```python
from build123d import *

# Parameters (mm, degrees)
SKETCH1_W               = 50
SKETCH1_H               = 95
BOSS_EXTRUDE1_DEPTH     = 4.5
SKETCH2_R               = 0.5
CUT_EXTRUDE1_DEPTH      = 108.448825028
SKETCH3_W               = 2
SKETCH3_H               = 2.25
CUT_EXTRUDE2_DEPTH      = 108.448825028
SKETCH5_R               = 2.5
BOSS_EXTRUDE2_DEPTH     = 2
SKETCH6_R               = 1.5
CUT_EXTRUDE3_DEPTH      = 108.551150621
FILLET1_R               = 4
SKETCH8_W               = 5.5
SKETCH8_H               = 30
CUT_EXTRUDE4_DEPTH      = 3
SKETCH10_W              = 2
SKETCH10_H              = 2.25
CUT_EXTRUDE5_DEPTH      = 4.5
FILLET2_R               = 1
SKETCH11_W              = 8
SKETCH11_H              = 2
BOSS_EXTRUDE3_DEPTH     = 8
CUT_EXTRUDE6_DEPTH      = 109.079831606
CUT_EXTRUDE6_DEPTH_BACK = 109.079831606
SKETCH12_R              = 1.7
FILLET3_R               = 2


with BuildPart() as part:
    # Sketch1 → Boss-Extrude1 (new body)
    with BuildSketch(Plane(origin=(0, 0, 0), x_dir=(0, 1, 0), z_dir=(0, 0, 1))):
        with Locations((25, 47.5)):
            Rectangle(SKETCH1_W, SKETCH1_H)
    extrude(amount=BOSS_EXTRUDE1_DEPTH)

    # Sketch2 → Cut-Extrude1 (cut, through all)
    with BuildSketch(Plane.XY.offset(4.5)):
        with Locations((-60, 25)):
            Circle(SKETCH2_R)
    extrude(amount=-CUT_EXTRUDE1_DEPTH, mode=Mode.SUBTRACT)

    # Sketch3 → Cut-Extrude2 (cut, through all)
    with BuildSketch(Plane(origin=(-95, 0, 0), x_dir=(0, -1, 0), z_dir=(-1, 0, 0))):
        with Locations((-49, 1.125)):
            Rectangle(SKETCH3_W, SKETCH3_H)
        with Locations((-1, 1.125)):
            Rectangle(SKETCH3_W, SKETCH3_H)
    extrude(amount=-CUT_EXTRUDE2_DEPTH, mode=Mode.SUBTRACT)

    # Sketch5 → Boss-Extrude2 (add)
    with BuildSketch(Plane.XY.offset(4.5)):
        with Locations(Location((-60, 25, 0), (0, 0, 180))):
            Circle(SKETCH5_R)
    extrude(amount=BOSS_EXTRUDE2_DEPTH)

    # Sketch6 → Cut-Extrude3 (cut, through all)
    with BuildSketch(Plane.XY.offset(6.5)):
        with Locations((-60, 25)):
            Circle(SKETCH6_R)
    extrude(amount=-CUT_EXTRUDE3_DEPTH, mode=Mode.SUBTRACT)

    # Fillet1
    # the kernel refuses this fillet: 4 mm, written as the material it adds along each edge
    with BuildSketch(Plane(origin=(-60, 25, 4.5), x_dir=(-1, 0, 0), z_dir=(0, 1, 0))) as fillet1_piece_1:
        with BuildLine():
            CenterArc((5.964101615, 4), FILLET1_R, 210, 60)
            Line((2.5, 2), (2.430717968, 1.96))
            ThreePointArc((2.430717968, 1.96), (2.42, 1), (2.42, 0))
            Line((2.42, 0), (2.5, -0.08))
            Line((2.5, -0.08), (5.964101615, -0.08))
            Line((5.964101615, -0.08), (5.964101615, 0))
        make_face()
    revolve(axis=Axis((-60, 25, 4.5), (0, 0, 1)))

    # Sketch8 → Cut-Extrude4 (cut)
    with BuildSketch(Plane(origin=(0, 0, 0), x_dir=(1, 0, 0), z_dir=(0, 0, -1))):
        with Locations((-60, -35)):
            Rectangle(SKETCH8_W, SKETCH8_H)
    extrude(amount=-CUT_EXTRUDE4_DEPTH, mode=Mode.SUBTRACT)

    # Sketch10 → Cut-Extrude5 (cut)
    with BuildSketch(Plane(origin=(-95, 0, 0), x_dir=(0, -1, 0), z_dir=(-1, 0, 0))):
        with Locations((-49, 3.375)):
            Rectangle(SKETCH10_W, SKETCH10_H)
        with Locations((-1, 3.375)):
            Rectangle(SKETCH10_W, SKETCH10_H)
    extrude(amount=-CUT_EXTRUDE5_DEPTH, mode=Mode.SUBTRACT)

    # Fillet2
    fillet2_edges = [part.edges().sort_by_distance(p)[0] for p in [
        (-95, 25, 0),
        (-95, 48, 2.25),
        (-95, 2, 2.25),
    ]]
    fillet(fillet2_edges, radius=FILLET2_R)

    # Sketch11 → Boss-Extrude3 (add)
    with BuildSketch(Plane.XY.offset(4.5)):
        with Locations((-4, 49)):
            Rectangle(SKETCH11_W, SKETCH11_H)
        with Locations((-4, 1)):
            Rectangle(SKETCH11_W, SKETCH11_H)
    extrude(amount=BOSS_EXTRUDE3_DEPTH)

    # Sketch12 → Cut-Extrude6 (cut, two sides: drawn at the far end of the back side and taken through both)
    with BuildSketch(Plane(origin=(0, 50, 0), x_dir=(-1, 0, 0), z_dir=(0, 1, 0)).offset(-CUT_EXTRUDE6_DEPTH_BACK)):
        with Locations((4, 8.5)):
            Circle(SKETCH12_R)
    extrude(amount=CUT_EXTRUDE6_DEPTH + CUT_EXTRUDE6_DEPTH_BACK, mode=Mode.SUBTRACT)

    # Fillet3
    fillet3_edges = [part.edges().sort_by_distance(p)[0] for p in [
        (-8, 49, 4.5),
        (0, 49, 12.5),
        (-8, 49, 12.5),
        (-8, 1, 4.5),
        (0, 1, 12.5),
        (-8, 1, 12.5),
    ]]
    fillet(fillet3_edges, radius=FILLET3_R)


solid = part.part
```
Input: part model. Units: mm. Frame: model coordinates. A direction names the side the tool comes from. Round coordinates to 2 decimals unless told otherwise and drop trailing zeros. Loops run counter-clockwise (first coordinate to the right, second up) from the corner with the lowest first, then second, coordinate; pieces in that order, holes last. Notation, with made-up numbers: (58, 40) - (110, 40) arc R21 cw to (110, 60) - close; hole circle Ø10 at (-30.5, 56.25). An arc over 180 degrees is marked (long way). One line per item, written item: value. Start each with the question number.
(1) Ray query, line 1 (Z direction, x = -4, y = 0.5); line 2 (X direction, y = 1.3, z = 8.5); line 3 (Z direction, x = -74.5, y = 29). Return the intervals inside material, ascending. Write a range as [from, to].
(2) Section A-A, the plane x = -4. Return loops of the section in (y, z), plus the area to 3 significant figures.
(3) Section C-C, the plane y = 25. Return loops of the section in (x, z), plus the area to 3 significant figures.
(4) Access query for faces 5 (the flat face through (-8, 49, 8)), 6 (the flat face through (-5.1, 2, 6.7)), 7 (the flat face through (-39, 50, 4)), 8 (the flat face through (-60, 20, 1)), 9 (the flat face through (-90.5, 49, 3)). Directions: +Z, -Z, +X, -X, +Y, -Y. A direction counts if a zero-diameter tool reaches every point of the face in a straight line with its end or side. Return the directions, or none.
(5) Draft query along X for faces 1 (the flat face through (-57.25, 35, 1)), 2 (the flat face through (-62.75, 35, 1)), 3 (the flat face through (-29, 48, 1)), 4 (the cylindrical face through (-0.57, 1.01, 11.9)). Return one class per face: +X half, -X half, draft (parallel to the pull), parting line (faces both ways), or undercut.
(6) Section B-B, the plane z = 8.5. Return loops of the section in (x, y), plus the area to 3 significant figures.
(7) Section D-D, the plane x = -71.5. Return loops of the section in (y, z).
(8) Contact query for flat-ended pins moving along their axis: P1, Ø1, axis at y = 49, z = 3.5, coming from the -X side; P2, Ø0.7, axis at x = -40.5, z = 1.5, coming from the +Y side; P3, Ø2, axis at y = 1, z = 9, coming from the -X side. Output: stop coordinate, or through.
Results below:
1. line 1: [2.25, 6.8], [10.2, 12.5]
1. line 2: [-8, -5.7], [-2.3, 0]
1. line 3: [0, 4.5]
2. outline: (0, 2.25) - (2, 2.25) - (2, 0) - (48, 0) - (48, 2.25) - (50, 2.25) - (50, 6.8) - (48, 6.8) - (48, 4.5) - (2, 4.5) - (2, 6.8) - (0, 6.8) - close; (0, 10.2) - (2, 10.2) - (2, 12.5) - (0, 12.5) - close; (48, 10.2) - (50, 10.2) - (50, 12.5) - (48, 12.5) - close
2. area: 234 mm^2
3. outline: (-95, 1) arc R1 ccw to (-94, 0) - (-62.75, 0) - (-62.75, 3) - (-61.5, 3) - (-61.5, 6.5) - (-62.5, 6.5) arc R4 cw to (-65.96, 4.5) - (-95, 4.5) - close; (-58.5, 3) - (-57.25, 3) - (-57.25, 0) - (0, 0) - (0, 4.5) - (-54.04, 4.5) arc R4 cw to (-57.5, 6.5) - (-58.5, 6.5) - close
3. area: 414 mm^2
4. face 5: +Z, -X, +Y, -Y
4. face 6: +Z, +X, -X
4. face 7: +Z, -Z, +X, -X, +Y
4. face 8: -Z, +Y
4. face 9: +Z, -Z, -X, +Y
5. face 1: undercut
5. face 2: undercut
5. face 3: draft
5. face 4: +X half
6. outline: (-8, 0) - (-5.7, 0) - (-5.7, 2) - (-8, 2) - close; (-8, 48) - (-5.7, 48) - (-5.7, 50) - (-8, 50) - close; (-2.3, 0) - (0, 0) - (0, 2) - (-2.3, 2) - close; (-2.3, 48) - (0, 48) - (0, 50) - (-2.3, 50) - close
6. area: 18.4 mm^2
7. outline: (0, 2.25) - (2, 2.25) - (2, 0) - (48, 0) - (48, 2.25) - (50, 2.25) - (50, 4.5) - (0, 4.5) - close
8. P1: x = -90.5
8. P2: y = 48
8. P3: x = -8
